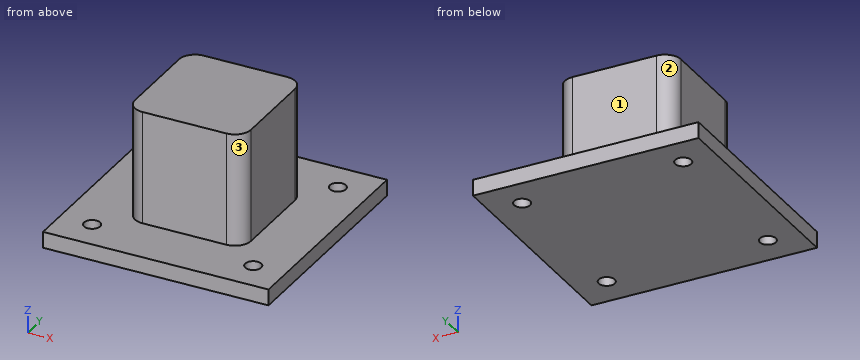
from build123d import *

# Parameters (mm, degrees)
F0_W     = 70
F0_H     = 70
F1_DEPTH = 5
F2_D     = 5
F3_W     = 36
F3_H     = 36
F4_DEPTH = 35
F5_R     = 5


# Not quite as in the source:
# - a feature names something its author has since deleted; it is built from what else it names


with BuildPart() as f1:
    # F0 (on Top) → F1 (new body)
    with BuildSketch(Plane.XY):
        Rectangle(F0_W, F0_H)
    extrude(amount=F1_DEPTH)

    # F2 (through all)
    with Locations(Plane(origin=(0, 0, 0), x_dir=(1, 0, 0), z_dir=(0, 0, -1))):
        with Locations((-25, -25), (25, -25), (25, 25), (-25, 25)):
            Hole(F2_D / 2)

    # F3 (on face) → F4 (join)
    with BuildSketch(Plane.XY.offset(5)):
        Rectangle(F3_W, F3_H)
    extrude(amount=F4_DEPTH)

    # F5
    f5_edges = [f1.edges().sort_by_distance(p)[0] for p in [
        (-18, 18, 22.5),
        (-18, -18, 22.5),
        (18, -18, 22.5),
        (18, 18, 22.5),
    ]]
    fillet(f5_edges, radius=F5_R)


solid = f1.part
Geometry check sheet. Reference: the model listing, model coordinates, mm. Face numbers are marked on the shaded views. A direction names the side the tool comes from. Round coordinates to 2 decimals unless told otherwise and drop trailing zeros. Order: outer loops, then holes, each group sorted by start corner. A loop starts at its lowest first (then second) coordinate and runs counter-clockwise, first axis right, second up. Notation, with made-up numbers: M -5.75,-36 L 40.25,-36 A27 cw 40.25,3 Z; hole C 71,-21.5 d2. An arc over 180 degrees is marked long. Write each question's results on one line, items separated by ' | '. Start each with the question number.
1. Cross-section at D-D on x = -4. Record the boundary of the cut face in (y, z), plus the area to 3 significant figures.
2. Go/stop test with flat-tipped pins: P1, Ø4, axis at x = -3.5, z = 16, coming from the +Y side; P2, Ø3, axis at y = 5.5, z = 15, coming from the -X side; P3, Ø1.5, axis at x = -21.5, y = -9.5, coming from the +Z side. Record where each tip stops, or that it passes through.
3. Material ranges on L1, parallel to X at y = -25, z = 1; L2, parallel to Z at x = 30, y = 28, recorded low to high. Write a range as from..to.
4. Cross-section at A-A on x = -25. Record the boundary of the cut face in (y, z).
5. Set-up check for the marked faces 1, 2 and 3: record each of +Z, -Z, +X, -X, +Y, -Y from which the full face is reachable in a straight line by a thin tool's end or side.
6. Cross-section at C-C on z = 11.5. Record the boundary of the cut face in (x, y), plus the area to 3 significant figures.
Resolved:
1) outline: M -35,0 L 35,0 L 35,5 L 18,5 L 18,40 L -18,40 L -18,5 L -35,5 Z | area: 1,610 mm2
2) P1: y = 18 | P2: x = -18 | P3: z = 5
3) L1: -35..-27.5, -22.5..22.5, 27.5..35 | L2: 0..5
4) outline: M -35,0 L -27.5,0 L -27.5,5 L -35,5 Z; M -22.5,0 L 22.5,0 L 22.5,5 L -22.5,5 Z; M 27.5,0 L 35,0 L 35,5 L 27.5,5 Z
5) face 1: +Z, +X, -X, +Y | face 2: +Z, -X, +Y | face 3: +Z, +X, -Y
6) outline: M -18,-13 A5 ccw -13,-18 L 13,-18 A5 ccw 18,-13 L 18,13 A5 ccw 13,18 L -13,18 A5 ccw -18,13 Z | area: 1,270 mm2
